Design review of the part built by this model. Coordinates are the model's own, in mm. A direction names the side the tool comes from. Give positions to 0.01 mm unless a question says otherwise; leave off trailing zeros. Loops run counter-clockwise (first coordinate to the right, second up) from the corner with the lowest first, then second, coordinate; pieces in that order, holes last. Notation, with made-up numbers: (26.25, 56) -> (83.25, 56) arc R31 ccw to (83.25, 85) -> close; hole circle Ø6 at (-17.75, 19). An arc over 180 degrees is marked (long way). Use a Markdown table: item, result. Add a question column.
1. Add section D-D (z = 8.5). State the section outline as (x, y) points, and give its area (3 significant figures).
2. Add section C-C (x = 157.5). State the section outline as (y, z) points, and give its area (3 significant figures).
3. Add section A-A (z = 55.5). State the section outline as (x, y) points.
4. For faces 4 (the flat face through (112, 79, 41)), 5 (the flat face through (20, 0, 33)), 6 (the flat face through (107, 195, 36)), list the 3-axis set-ups (+Z, -Z, +X, -X, +Y, -Y) from which the entire face can be reached by the end or side of a thin tool; tool diameter is ignored.
5. For pin 1 Ø4 at (y, z) = (172, 31) entering from -X; pin 2 Ø3 at (x, y) = (10.5, 70.5) entering from +Z; pin 3 Ø3 at (x, y) = (28, 24) entering from +Z; pin 4 Ø6 at (y, z) = (71.5, 40) entering from +X, all flat-tipped, find the tip position at first contact; note any pin that passes through.
6. Add section B-B (y = 180). State the section outline as (x, z) points.
7. Draft analysis for pull direction X (two halves, no side actions). For faces 1 (the flat face through (121, 81, 33)), 2 (the flat face through (0, 99, 33)), 3 (the flat face through (194, 180, 62)), state which applies: pulls with the +X half, pulls with the -X half, needs draft (parallel to the pull), parting line crosses it, or undercut.
8. To check wall thickness, follow line 1 (Y direction, x = 27.5, z = 16.5); line 2 (Y direction, x = 10, z = 20); line 3 (X direction, y = 72.5, z = 30). State the ranges of each line that lie inside material, in increasing order.
```python
from build123d import *

# Parameters (mm, degrees)
ESTRUSIONE_ESTRUSIONE1_DEPTH  = 70
SVUOTA1_T                     = -3
SCHIZZO5_W                    = 4
SCHIZZO5_H                    = 200
TAGLIO_ESTRUSIONE1_DEPTH      = 1
TAGLIO_ESTRUSIONE1_DEPTH_BACK = 201
ESTRUSIONE_ESTRUSIONE4_DEPTH  = 38
SCHIZZO8_R                    = 2
TAGLIO_ESTRUSIONE2_DEPTH      = 30
SCHIZZO11_W                   = 160
SCHIZZO11_H                   = 5
ESTRUSIONE_ESTRUSIONE7_DEPTH  = 5
ESTRUSIONE_ESTRUSIONE8_DEPTH  = 62
ESTRUSIONE_ESTRUSIONE9_DEPTH  = 2


with BuildPart() as part:
    # Schizzo2 → Estrusione-Estrusione1 (new body)
    with BuildSketch(Plane.XY):
        Polygon((0, 0), (0, 200), (200, 200), (200, 160), (40, 0), align=None)
    extrude(amount=ESTRUSIONE_ESTRUSIONE1_DEPTH)

    # Svuota1
    svuota1_openings = [part.faces().sort_by_distance(p)[0] for p in [
        (88, 112, 70),
    ]]
    offset(amount=SVUOTA1_T, openings=svuota1_openings, kind=Kind.INTERSECTION)

    # Schizzo5 → Taglio-Estrusione1 (cut, two sides)
    with BuildSketch(Plane(origin=(200, 0, 0), x_dir=(0, 0, -1), z_dir=(1, 0, 0))) as taglio_estrusione1_sk:
        with Locations((-68, 100)):
            Rectangle(SCHIZZO5_W, SCHIZZO5_H)
    extrude(amount=TAGLIO_ESTRUSIONE1_DEPTH, mode=Mode.SUBTRACT)
    extrude(taglio_estrusione1_sk.sketch, amount=-TAGLIO_ESTRUSIONE1_DEPTH_BACK, mode=Mode.SUBTRACT)

    # Schizzo7 → Estrusione-Estrusione4 (add)
    with BuildSketch(Plane.XY.offset(41)):
        with BuildLine():
            Line((3, 170), (3, 131.842431943))
            ThreePointArc((3, 131.842431943), (17, 150.921215972), (3, 170))
        make_face()
        with BuildLine():
            Line((3, 90), (3, 51.842431943))
            ThreePointArc((3, 51.842431943), (17, 70.921215972), (3, 90))
        make_face()
    extrude(amount=-ESTRUSIONE_ESTRUSIONE4_DEPTH)

    # Schizzo8 → Taglio-Estrusione2 (cut)
    with BuildSketch(Plane.XY.offset(41)):
        with Locations((10, 150.921215972)):
            Circle(SCHIZZO8_R)
        with Locations((10, 70.921215972)):
            Circle(SCHIZZO8_R)
    extrude(amount=-TAGLIO_ESTRUSIONE2_DEPTH, mode=Mode.SUBTRACT)

    # Schizzo11 → Estrusione-Estrusione7 (add)
    with BuildSketch(Plane.XY.offset(41)):
        with Locations((108, 194.5)):
            Rectangle(SCHIZZO11_W, SCHIZZO11_H)
        Polygon((169.572113832, 133.81475452), (56.435028843, 20.67766953), (52.899494937, 24.213203436), (166.036579926, 137.350288425), align=None)
    extrude(amount=-ESTRUSIONE_ESTRUSIONE7_DEPTH)

    # Schizzo12 → Estrusione-Estrusione8 (add)
    with BuildSketch(Plane.XY.offset(62)):
        with BuildLine():
            Line((193, 184), (197, 184))
            Line((197, 184), (197, 176))
            Line((197, 176), (193, 176))
            ThreePointArc((193, 176), (189, 180), (193, 184))
        make_face()
    extrude(amount=-ESTRUSIONE_ESTRUSIONE8_DEPTH)

    # Schizzo13 → Estrusione-Estrusione9 (add)
    with BuildSketch(Plane.XY.offset(62)):
        with BuildLine():
            Line((193, 177), (196, 177))
            Line((196, 177), (197, 177))
            Line((197, 177), (197, 176))
            Line((197, 176), (193, 176))
            ThreePointArc((193, 176), (189, 180), (193, 184))
            Line((193, 184), (197, 184))
            Line((197, 184), (197, 183))
            Line((197, 183), (193, 183))
            ThreePointArc((193, 183), (190, 180), (193, 177))
        make_face()
    extrude(amount=ESTRUSIONE_ESTRUSIONE9_DEPTH)


solid = part.part
```
Taken from the geometry:
| question | item | result |
|---|---|---|
| 1 | outline | (0, 0) -> (40, 0) -> (200, 160) -> (200, 200) -> (0, 200) -> close; hole (3, 3) -> (38.76, 3) -> (197, 161.24) -> (197, 176) -> (193, 176) arc R4 cw to (193, 184) -> (197, 184) -> (197, 197) -> (3, 197) -> (3, 170) arc R20 cw to (3, 131.84) -> (3, 90) arc R20 cw to (3, 51.84) -> close |
| 1 | area | 2,930 mm^2 |
| 2 | outline | (117.5, 0) -> (200, 0) -> (200, 66) -> (197, 66) -> (197, 41) -> (192, 41) -> (192, 36) -> (197, 36) -> (197, 3) -> (121.74, 3) -> (121.74, 36) -> (128.81, 36) -> (128.81, 41) -> (121.74, 41) -> (121.74, 66) -> (117.5, 66) -> close |
| 2 | area | 764 mm^2 |
| 3 | outline | (0, 0) -> (40, 0) -> (200, 160) -> (200, 200) -> (0, 200) -> close; hole (3, 3) -> (38.76, 3) -> (197, 161.24) -> (197, 176) -> (193, 176) arc R4 cw to (193, 184) -> (197, 184) -> (197, 197) -> (3, 197) -> close |
| 4 | face 4 | +Z |
| 4 | face 5 | +Z, -Z, +X, -X, -Y |
| 4 | face 6 | none |
| 5 | pin 1 | stops at x = 0 |
| 5 | pin 2 | stops at z = 41 |
| 5 | pin 3 | stops at z = 3 |
| 5 | pin 4 | stops at x = 114.5 |
| 6 | outline | (0, 0) -> (200, 0) -> (200, 66) -> (197, 66) -> (197, 62) -> (190, 62) -> (190, 64) -> (189, 64) -> (189, 3) -> (3, 3) -> (3, 66) -> (0, 66) -> close |
| 7 | face 1 | pulls with the +X half |
| 7 | face 2 | pulls with the -X half |
| 7 | face 3 | undercut |
| 8 | line 1 | y = 0 to 3, 197 to 200 |
| 8 | line 2 | y = 0 to 3, 55.72 to 68.92, 72.92 to 86.12, 135.72 to 148.92, 152.92 to 166.12, 197 to 200 |
| 8 | line 3 | x = 0 to 8.77, 11.23 to 16.94, 108.26 to 112.5 |
